Part model, mm, in its own coordinate system. A direction names the side the tool comes from. Round coordinates to 2 decimals unless told otherwise and drop trailing zeros. Write each loop counter-clockwise with the first axis right and the second up, starting at its lowest first coordinate (ties: lowest second). Pieces come first, ordered by that corner, then holes. Notation, with made-up numbers: M -22,-31 L 33,-31 A23 cw 33,-17 Z; hole C -31,53 d3. An arc over 180 degrees is marked long. Use one line per item in the form item = value. Start each with the question number.
Item 1: Probe L1, parallel to Y at x = 4, z = 3.55; L2, parallel to X at y = -5.5, z = 1.2; L3, parallel to Z at x = 11, y = -5. List the from-to ranges inside material, lowest first.
Item 2: Flat gauge pins, fed straight in: pin 1 Ø2 at (x, y) = (-4, -3.5) entering from -Z; pin 2 Ø5 at (x, y) = (7, 1.5) entering from -Z. Where does each tip first touch, or does it go through?
Item 3: Cut at C-C, the plane x = 7.62. Give the cut face in (y, z), then the cut area to 3 significant figures.
Item 4: Mould opens along X. For faces 4 (the face through (13.774, 2.903, 4.141)), 5 (the face through (-12, 4, 5.029)) say: +X half, -X half, draft (parallel to the pull), parting line (faces both ways), or undercut.
Item 5: Cut at A-A, the plane z = 4. Give the cut face in (x, y).
Item 6: Cut at D-D, the plane x = -6. Give the cut face in (y, z).
Item 7: Which spindle directions (+Z, -Z, +X, -X, +Y, -Y) get a long thin tool onto all of the face, cutting with end or side? Do faces 1 (the face through (6.912, 3.186, 1.001)), 2 (the face through (-4, -4, 5.029)), 3 (the face through (1.881, 2.353, 4.141)). Say none if no direction does.
from build123d import *

# Parameters (mm, degrees)
F0_W      = 31.8516
F0_H      = 15.8496
F1_DEPTH  = 3.2766
F2_T      = -1.524
F3_R      = 3.2639
F4_DEPTH  = 1.524
F5_R      = 2.4765
F8_DEPTH  = 1.524
F6_R      = 2.4765
F9_DEPTH  = 1.524
F7_R      = 2.4765
F10_DEPTH = 1.524
F11_R     = 2.4384
F12_DEPTH = 1.7526
F13_R     = 1.2954
F14_DEPTH = 1.778


with BuildPart() as f1:
    # F0 (on Top) → F1 (new body)
    with BuildSketch(Plane.XY):
        Rectangle(F0_W, F0_H)
    extrude(amount=F1_DEPTH)

    # F2
    f2_openings = [f1.faces().sort_by_distance(p)[0] for p in [
        (0, 0, 0),
    ]]
    offset(amount=F2_T, openings=f2_openings)

    # F3 (on face) → F4 (join)
    with BuildSketch(Plane(origin=(0, 0, 1.7526), x_dir=(1, 0, 0), z_dir=(0, 0, -1))):
        Circle(F3_R)
        with Locations((-7.62, 0)):
            Circle(F3_R)
        with Locations((7.62, 0)):
            Circle(F3_R)
    extrude(amount=F4_DEPTH)

    # F5 (on face) → F8 (cut)
    with BuildSketch(Plane(origin=(0, 0, 0.2286), x_dir=(1, 0, 0), z_dir=(0, 0, -1))):
        Circle(F5_R)
    extrude(amount=-F8_DEPTH, mode=Mode.SUBTRACT)

    # F6 (on face) → F9 (cut)
    with BuildSketch(Plane(origin=(0, 0, 0.2286), x_dir=(1, 0, 0), z_dir=(0, 0, -1))):
        with Locations((-7.62, 0)):
            Circle(F6_R)
    extrude(amount=-F9_DEPTH, mode=Mode.SUBTRACT)

    # F7 (on face) → F10 (cut)
    with BuildSketch(Plane(origin=(0, 0, 0.2286), x_dir=(1, 0, 0), z_dir=(0, 0, -1))):
        with Locations((7.62, 0)):
            Circle(F7_R)
    extrude(amount=-F10_DEPTH, mode=Mode.SUBTRACT)

    # F11 (on face) → F12 (join)
    with BuildSketch(Plane.XY.offset(3.2766)):
        with Locations((-11.55889, 3.837082)):
            Circle(F11_R)
        with Locations((-3.853228, 3.837082)):
            Circle(F11_R)
        with Locations((3.815653, 3.837082)):
            Circle(F11_R)
        with Locations((11.521315, 3.837082)):
            Circle(F11_R)
        with Locations((11.521315, -3.831711)):
            Circle(F11_R)
        with Locations((3.815653, -3.831711)):
            Circle(F11_R)
        with Locations((-3.853228, -3.831711)):
            Circle(F11_R)
        with Locations((-11.55889, -3.831711)):
            Circle(F11_R)
    extrude(amount=F12_DEPTH)

    # F13 (on face) → F14 (cut)
    with BuildSketch(Plane(origin=(0, 0, 0), x_dir=(1, 0, 0), z_dir=(0, 0, -1))):
        with Locations((-3.98145, 3.9624)):
            Circle(F13_R)
        with Locations((-11.94435, 3.9624)):
            Circle(F13_R)
        with Locations((-11.94435, -3.9624)):
            Circle(F13_R)
        with Locations((-3.98145, -3.9624)):
            Circle(F13_R)
        with Locations((3.98145, -3.9624)):
            Circle(F13_R)
        with Locations((11.94435, -3.9624)):
            Circle(F13_R)
        with Locations((11.94435, 3.9624)):
            Circle(F13_R)
        with Locations((3.98145, 3.9624)):
            Circle(F13_R)
    extrude(amount=-F14_DEPTH, mode=Mode.SUBTRACT)


solid = f1.part
Model answer:
q1.L1 = -6.26 to -1.4, 1.41 to 6.27
q1.L2 = -15.93 to -14.4, 14.4 to 15.93
q1.L3 = 1.75 to 5.03
q2.pin_1 = 1.75
q2.pin_2 = 0.23
q3.outline = M -7.92,0 L -6.4,0 L -6.4,1.75 L -3.26,1.75 L -3.26,0.23 L -2.48,0.23 L -2.48,1.75 L 2.48,1.75 L 2.48,0.23 L 3.26,0.23 L 3.26,1.75 L 6.4,1.75 L 6.4,0 L 7.92,0 L 7.92,3.28 L -7.92,3.28 Z
q3.area = 31.9 mm²
q4.face_4 = undercut
q4.face_5 = draft
q5.outline = C -11.56,-3.83 d4.88; C -11.56,3.84 d4.88; C -3.85,-3.83 d4.88; C -3.85,3.84 d4.88; C 3.82,-3.83 d4.88; C 3.82,3.84 d4.88; C 11.52,-3.83 d4.88; C 11.52,3.84 d4.88
q6.outline = M -7.92,0 L -6.4,0 L -6.4,1.75 L -2.83,1.75 L -2.83,0.23 L -1.87,0.23 L -1.87,1.75 L 1.87,1.75 L 1.87,0.23 L 2.83,0.23 L 2.83,1.75 L 6.4,1.75 L 6.4,0 L 7.92,0 L 7.92,3.28 L 4.99,3.28 L 4.99,5.03 L 2.68,5.03 L 2.68,3.28 L -2.68,3.28 L -2.68,5.03 L -4.99,5.03 L -4.99,3.28 L -7.92,3.28 Z
q7.face_1 = -Z
q7.face_2 = +Z, +X, -X, +Y, -Y
q7.face_3 = +Z
